Build history of the part. All positions in model axes, mm. A direction names the side the tool comes from. Round coordinates to 2 decimals unless told otherwise and drop trailing zeros. Loops run counter-clockwise (first coordinate to the right, second up) from the corner with the lowest first, then second, coordinate; pieces in that order, holes last. Notation, with made-up numbers: (71.5, 72.5) - (82.5, 72.5) arc R20 ccw to (82.5, 86.5) - close; hole circle Ø1 at (81.5, 72.25). An arc over 180 degrees is marked (long way). Use one line per item in the form item = value. Start each with the question number.
Q1. Drill centre line: line 1 (Y direction, x = 29.5, z = 0.75). Where is it in solid material? Low to high.
Q2. Saw through at A-A (y = 0). Give the cut face in (x, z).
Q3. Saw through at B-B (z = 5). Give the cut face in (x, y).
Q4. Saw through at C-C (x = 35.5). Give the cut face in (y, z), then the cut area to 3 significant figures.
Q5. 3-axis set-ups, long thin cutter, end or side, ignore diameter. For faces 1 (the face through (44.57, 0.39, 1.25)), 2 (the face through (42, -7, 2.54)): which of +Z, -Z, +X, -X, +Y, -Y reach the whole face in a straight line?
Q6. Mould opens along Y. For faces 3 (the face through (-1, 76.2, 3)), 4 (the face through (-1, -76.2, 3)), 5 (the face through (46.255, -4.329, 4.472)), 6 (the face through (-1, 1, 6.35)) say: released by +Y, released by -Y, zero draft, split by the parting line, or undercut.
```python
from build123d import *

# Parameters (mm, degrees)
F0_W           = 101.6
F0_H           = 152.4
F1_DEPTH       = 6.35
F3_D           = 17.526
F3_CBORE_D     = 22.606
F3_CBORE_DEPTH = 3.81


with BuildPart() as f1:
    # F0 (on Top) → F1 (new body)
    with BuildSketch(Plane.XY):
        Rectangle(F0_W, F0_H)
    extrude(amount=F1_DEPTH)

    # F3 (through all)
    with Locations(Plane.XY.offset(6.35)):
        with Locations((35.814, 0)):
            CounterBoreHole(F3_D / 2, F3_CBORE_D / 2, F3_CBORE_DEPTH)


solid = f1.part
```
Report:
q1.line_1 = -76.2 to -6.08, 6.08 to 76.2
q2.outline = (-50.8, 0) - (27.05, 0) - (27.05, 2.54) - (24.51, 2.54) - (24.51, 6.35) - (-50.8, 6.35) - close; (44.58, 0) - (50.8, 0) - (50.8, 6.35) - (47.12, 6.35) - (47.12, 2.54) - (44.58, 2.54) - close
q3.outline = (-50.8, -76.2) - (50.8, -76.2) - (50.8, 76.2) - (-50.8, 76.2) - close; hole circle Ø22.61 at (35.81, 0)
q4.outline = (-76.2, 0) - (-8.76, 0) - (-8.76, 2.54) - (-11.3, 2.54) - (-11.3, 6.35) - (-76.2, 6.35) - close; (8.76, 0) - (76.2, 0) - (76.2, 6.35) - (11.3, 6.35) - (11.3, 2.54) - (8.76, 2.54) - close
q4.area = 837 mm²
q5.face_1 = +Z, -Z
q5.face_2 = +Z
q6.face_3 = released by +Y
q6.face_4 = released by -Y
q6.face_5 = undercut
q6.face_6 = zero draft
